CAD build for the part. Positions are in the model's coordinates, mm. A direction names the side the tool comes from. Give positions to 0.01 mm unless a question says otherwise; leave off trailing zeros. Order: outer loops, then holes, each group sorted by start corner. A loop starts at its lowest first (then second) coordinate and runs counter-clockwise, first axis right, second up.
```python
from build123d import *

# Parameters (mm, degrees)
BOSS_EXTRUDE1_DEPTH = 13.462
SKETCH2_R           = 6.858
CUT_EXTRUDE1_DEPTH  = 12.954
SKETCH3_R           = 5.1435
BOSS_EXTRUDE2_DEPTH = 13.462
SKETCH4_R           = 2.794
CUT_EXTRUDE2_DEPTH  = 27.924


with BuildPart() as part:
    # Sketch1 → Boss-Extrude1 (new body)
    with BuildSketch(Plane(origin=(0, 0, 0), x_dir=(1, 0, 0), z_dir=(0, 1, 0))):
        Polygon((5.499261314, 9.525), (-5.499261314, 9.525), (-10.998522628, 0), (-5.499261314, -9.525), (5.499261314, -9.525), (10.998522628, 0), align=None)
    extrude(amount=-BOSS_EXTRUDE1_DEPTH)

    # Sketch2 → Cut-Extrude1 (cut)
    with BuildSketch(Plane(origin=(0, 0, 0), x_dir=(1, 0, 0), z_dir=(0, 1, 0))):
        Circle(SKETCH2_R)
    extrude(amount=-CUT_EXTRUDE1_DEPTH, mode=Mode.SUBTRACT)

    # Sketch3 → Boss-Extrude2 (add)
    with BuildSketch(Plane.XZ.offset(13.462)):
        Circle(SKETCH3_R)
    extrude(amount=BOSS_EXTRUDE2_DEPTH)

    # Sketch4 → Cut-Extrude2 (cut, through all)
    with BuildSketch(Plane.XZ.offset(26.924)):
        Circle(SKETCH4_R)
    extrude(amount=-CUT_EXTRUDE2_DEPTH, mode=Mode.SUBTRACT)


solid = part.part
```
Item 1: Slice it at D-D (y = -23). Give the cut face in (x, z), and give its area (3 significant figures).
Item 2: Slice it at A-A (x = 0). Give the cut face in (y, z) (1 decimal), and give its area (3 significant figures).
Item 3: Slice it at C-C (x = 6.25). Give the cut face in (y, z), and give its area (3 significant figures).
Item 4: Drop flat-ended pins along their axis: pin 1 Ø2 at (y, z) = (-9.5, 7) entering from -X; pin 2 Ø4 at (x, y) = (4, -23) entering from -Z; pin 3 Ø5 at (x, z) = (0, 0) entering from +Y; pin 4 Ø10 at (y, z) = (-10, 6.5) entering from +X. Give the stop position or say it passes through.
Item 5: Tool access for faces 5 (the face through (-0.67, -20.1, 5.1)), 6 (the face through (0, -7, -9.525)): list every direction of +Z, -Z, +X, -X, +Y, -Y with a clear straight run to the whole face (end or side of a thin tool).
Item 6: Slice it at B-B (y = -12.5). Give the cut face in (x, z) (3 decimals).
Item 7: Wall check: L1, parallel to Z at x = 0, y = -23.5; L2, parallel to Y at x = 3, z = -3.75; L3, parallel to Y at x = 1, z = 6.25. Give the ranges that are in metal, low to high.
Item 8: Two-plate mould, pull along Z, no slides. Class faces 1 (the face through (3, -12.954, 0)), 2 (the face through (8.21, -6.64, 4.83)), 3 (the face through (-1.487, -6.386, 6.695)), 4 (the face through (5, -13.462, -2)): released by +Z, released by -Z, zero draft, split by the parting line, or undercut.
A:
1. outline: circle Ø10.29 at (0, 0); hole circle Ø5.59 at (0, 0)
1. area: 58.6 mm2
2. outline: (-26.9, -5.1) - (-13.5, -5.1) - (-13.5, -9.5) - (0, -9.5) - (0, -6.9) - (-13, -6.9) - (-13, -2.8) - (-26.9, -2.8) - close; (-26.9, 2.8) - (-13, 2.8) - (-13, 6.9) - (0, 6.9) - (0, 9.5) - (-13.5, 9.5) - (-13.5, 5.1) - (-26.9, 5.1) - close
2. area: 139 mm2
3. outline: (-13.46, -8.22) - (0, -8.22) - (0, -2.82) - (-12.95, -2.82) - (-12.95, 2.82) - (0, 2.82) - (0, 8.22) - (-13.46, 8.22) - close
3. area: 148 mm2
4. pin 1: stops at x = -7.53
4. pin 2: stops at z = -4.74
4. pin 3: passes through
4. pin 4: stops at x = 10.13
5. face 5: -Y
5. face 6: -Z, +X, -X, +Y, -Y
6. outline: (-10.999, 0) - (-5.499, -9.525) - (5.499, -9.525) - (10.999, 0) - (5.499, 9.525) - (-5.499, 9.525) - close; hole circle Ø13.716 at (0, 0)
7. L1: z = -5.14 to -2.79, 2.79 to 5.14
7. L2: y = -26.92 to -12.95
7. L3: y = -13.46 to -12.95
8. face 1: undercut
8. face 2: released by +Z
8. face 3: undercut
8. face 4: zero draft
